Autodesk Inventor part; units mm, degrees
ref_plane "Work Plane1" through (0, 12.7, 0) normal (0, 1, 0) x (-1, 0, 0)
ref_plane "YZ Plane" through (0, 0, 0) normal (1, 0, 0) x (0, 1, 0)
ref_plane "XY Plane" through (0, 0, 0) normal (0, 0, 1) x (1, 0, 0)
sketch "Sketch2" plane through (0, 0, 0) normal (0, 0, 1) x (1, 0, 0)
  circle A0 centre (0, 0) radius 12.7
  dimension "d0" = 25.4
extrude "Extrusion1" add sketch "Sketch2" along normal blind 73.025
sketch "Sketch3" plane through (0, 0, 73.025) normal (0, 0, 1) x (1, 0, 0)
  arc A0 (-6.5485, -1.2541) -> (-6.4558, 1.6669) centre (0, 0) ccw
  circle A1 centre (0, 0) radius 12.7 construction
  line L0 (-12.7, 0) -> (12.7, 0) construction
  line L1 (-6.35, 0) -> (-4.7625, 1.5875) construction
  line L2 (-4.7625, -1.5875) -> (-6.35, 0) construction
  line L3 (-6.5485, -1.2541) -> (-5.1223, -1.2541)
  line L4 (-5.1223, -1.2541) -> (-5.1223, 1.6669)
  line L5 (-5.1223, 1.6669) -> (-6.4558, 1.6669)
  dimension "d3" = 13.335
  dimension "d22" = 2.921
  dimension "d23" = 1.3335
extrude "Extrusion2" cut sketch "Sketch3" against normal blind 25.4
sketch "Sketch4" plane through (0, 0, 0) normal (0, 0, -1) x (-1, 0, 0)
  circle A0 centre (0, 0) radius 3.175
  dimension "d10" = 6.35
extrude "Extrusion3" cut sketch "Sketch4" against normal through all
ref_plane "Work Plane1" through (0, 12.7, 0) normal (0, 1, 0) x (-1, 0, 0)
sketch "Sketch5" plane through (0, 12.7, 0) normal (0, 1, 0) x (-1, 0, 0)
  line L0 (-12.7, 0) -> (12.7, 0)
  point P0 (0, 0)
  point P1 (0, 9.525)
  dimension "d13" = 9.525
hole "Hole1" at (0, 12.7, 9.525) direction (0, -1, 0) diameter 2.6416 end through all
sketch "Sketch6" plane through (0, 12.7, 0) normal (0, 1, 0) x (-1, 0, 0)
  line L0 (12.7, 73.025) -> (-12.7, 73.025)
  point P0 (0, 0)
  point P1 (0, 63.5)
  dimension "d24" = 9.525
hole "Hole2" at (0, 12.7, 63.5) direction (0, -1, 0) diameter 2.6416 end through all
equation "\"d1\" = length"
equation "\"d3\" = shaftDiameter + shaftClearance"
equation "\"d22\" = keywayWidth"
equation "\"d23\" = keywayDepth"
equation "\"length\" = 73.025"
equation "\"shaftDiameter\" = 12.7"
equation "\"shaftClearance\" = 0.635"
equation "\"keywayWidth\" = 2.921"
equation "\"keywayDepth\" = 1.3335"
properties part number "ShaftToConnectPotToMotor" material "Aluminum 6061"
Check sheet for the modelled part. Datum: model origin and axes. Units: mm. A direction names the side the tool comes from. Give positions to 0.01 mm unless a question says otherwise; leave off trailing zeros. Loops run counter-clockwise (first coordinate to the right, second up) from the corner with the lowest first, then second, coordinate; pieces in that order, holes last. Notation, with made-up numbers: M 87,-33 L 121,-33 A13 cw 121,-16 Z; hole C 15,17 d7. An arc over 180 degrees is marked long. Answer in a Markdown table with one row per item.
1) Cross-section at C-C (z = 23.5). Enter the section's corners in (x, y) (3 decimals), plus the area to 3 significant figures.
Solutions:
| item | result |
|---|---|
| outline | C 0,0 d25.4; hole C 0,0 d6.35 |
| area | 475 mm^2 |
2) Cross-section at A-A (y = 0). Enter the section's corners in (x, z) (1 decimal), plus the area to 3 significant figures.
Solutions:
| item | result |
|---|---|
| outline | M -12.7,0 L -3.2,0 L -3.2,47.6 L -5.1,47.6 L -5.1,73 L -12.7,73 Z; M 3.2,0 L 12.7,0 L 12.7,73 L 6.7,73 L 6.7,47.6 L 3.2,47.6 Z |
| area | 1,250 mm^2 |
3) Depth check by flat-ended pin: pin 1 (5 mm diameter, centred on x = -4.5, z = 60, fed in from +Y); pin 2 (0.7 mm diameter, centred on x = -6, z = 64.5, fed in from -Y); pin 3 (3 mm diameter, centred on x = 2, z = 23.5, fed in from -Y). Enter the tip coordinate at first touch or a pass-through.
Solutions:
| item | result |
|---|---|
| pin 1 | stops at y = 12.54 |
| pin 2 | stops at y = -11.37 |
| pin 3 | stops at y = -12.69 |
4) Cross-section at D-D (z = 63.5). Enter the section's corners in (x, y), plus the area to 3 significant figures.
Solutions:
| item | result |
|---|---|
| outline | M -6.55,-1.25 L -5.12,-1.25 L -5.12,1.67 L -6.46,1.67 A6.67 cw -1.32,6.54 L -1.32,12.63 A12.7 ccw -1.32,-12.63 L -1.32,-6.54 A6.67 cw Z; M 1.32,-12.63 A12.7 ccw 1.32,12.63 L 1.32,6.54 A6.67 cw 1.32,-6.54 Z |
| area | 339 mm^2 |
5) Thickness scan on line 1 (Z direction, x = 0, y = 10.5) (3 decimals); line 2 (Y direction, x = -4.5, z = 52.5); line 3 (X direction, y = 10.75, z = 63.5). Record the ranges inside material, lowest first.
Solutions:
| item | result |
|---|---|
| line 1 | z = 0 to 8.204, 10.846 to 62.179, 64.821 to 73.025 |
| line 2 | y = -11.88 to -4.92, 4.92 to 11.88 |
| line 3 | x = -6.76 to -1.32, 1.32 to 6.76 |
6) Cross-section at B-B (x = 0). Enter the section's corners in (y, z) (3 decimals), plus the area to 3 significant figures.
Solutions:
| item | result |
|---|---|
| outline | M -12.7,0 L -3.175,0 L -3.175,8.204 L -12.7,8.204 Z; M -12.7,10.846 L -3.175,10.846 L -3.175,47.625 L -6.667,47.625 L -6.667,62.179 L -12.7,62.179 Z; M -12.7,64.821 L -6.667,64.821 L -6.667,73.025 L -12.7,73.025 Z; M 3.175,0 L 12.7,0 L 12.7,8.204 L 3.175,8.204 Z; M 3.175,10.846 L 12.7,10.846 L 12.7,62.179 L 6.668,62.179 L 6.668,47.625 L 3.175,47.625 Z; M 6.668,64.821 L 12.7,64.821 L 12.7,73.025 L 6.668,73.025 Z |
| area | 1,130 mm^2 |
7) Tool access check on faces 5 (the face through (-5.122, 0, 61)), 6 (the face through (-0.058, 7.725, 8.205)). Record the directions out of +Z, -Z, +X, -X, +Y, -Y that give a thin tool (end or side, any length) a straight path to the whole face; none if there is none.
Solutions:
| item | result |
|---|---|
| face 5 | +Z |
| face 6 | +Y, -Y |
8) Mould release check, pull along X, two halves, no side actions. Record for faces 1 (the face through (-6, -1.254, 61)), 2 (the face through (-0.058, -7.862, 8.205)), 3 (the face through (3, -3, 0)), 4 (the face through (-2.75, 12.4, 36)): released by +X, released by -X, zero draft, split by the parting line, or undercut.
Solutions:
| item | result |
|---|---|
| face 1 | undercut |
| face 2 | undercut |
| face 3 | zero draft |
| face 4 | split by the parting line |
